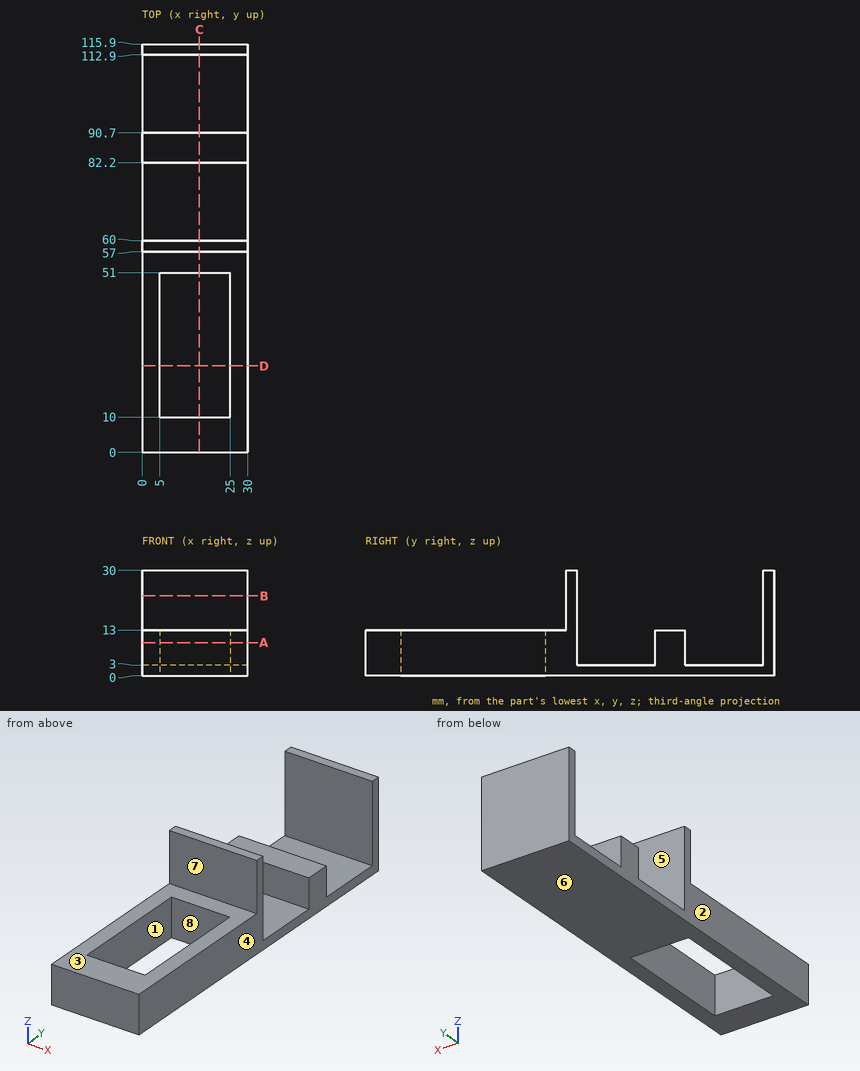
Geometry check sheet. Reference: drawing and pictorial views, mm from the part's lowest x, y, z. A direction names the side the tool comes from. Coordinates: 2 decimals unless noted, no trailing zeros. Order: outer loops, then holes, each group sorted by start corner. A loop starts at its lowest first (then second) coordinate and runs counter-clockwise, first axis right, second up.
Item 1: Section check C-C (x = 16.25). Enter the section's corners in (y, z).
Item 2: Scan lines: line 1 along Y through (x, z) = (19.75, 5.75); line 2 along Y through (x, z) = (27.5, 8); line 3 along Y through (x, z) = (19.75, 18.5). Record each from-to range of solid material in increasing order.
Item 3: Depth check by flat-ended pin: pin 1 (8 mm diameter, centred on x = 14, z = 18.5, fed in from -Y); pin 2 (6 mm diameter, centred on x = 7.5, y = 104.5, fed in from +Z); pin 3 (2.5 mm diameter, centred on x = 21, y = 85.5, fed in from +Z). Enter the tip coordinate at first touch or a pass-through.
Item 4: Section check A-A (z = 9.5). Enter the section's corners in (x, y), plus the area to 4 significant figures.
Item 5: Section check D-D (y = 24.5). Enter the section's corners in (x, z).
Item 6: Section check B-B (z = 22.75). Enter the section's corners in (x, y).
Item 7: Tool access check on the marked faces 5, 6, 7 and 8. Record the directions out of +Z, -Z, +X, -X, +Y, -Y that give a thin tool (end or side, any length) a straight path to the whole face; none if there is none.
Item 8: Mould release check, pull along X, two halves, no side actions. Record for the marked faces 1, 2, 3 and 4: released by +X, released by -X, zero draft, split by the parting line, or undercut.
Check sheet entries:
1. outline: (0, 0) - (10, 0) - (10, 13) - (0, 13) - close; (51, 0) - (115.9, 0) - (115.9, 30) - (112.9, 30) - (112.9, 3) - (90.7, 3) - (90.7, 13) - (82.2, 13) - (82.2, 3) - (60, 3) - (60, 30) - (57, 30) - (57, 13) - (51, 13) - close
2. line 1: y = 0 to 10, 51 to 60, 82.2 to 90.7, 112.9 to 115.9
2. line 2: y = 0 to 60, 82.2 to 90.7, 112.9 to 115.9
2. line 3: y = 57 to 60, 112.9 to 115.9
3. pin 1: stops at y = 57
3. pin 2: stops at z = 3
3. pin 3: stops at z = 13
4. outline: (0, 0) - (30, 0) - (30, 60) - (0, 60) - close; (0, 82.2) - (30, 82.2) - (30, 90.7) - (0, 90.7) - close; (0, 112.9) - (30, 112.9) - (30, 115.9) - (0, 115.9) - close; hole (5, 10) - (25, 10) - (25, 51) - (5, 51) - close
4. area: 1,325 mm2
5. outline: (0, 0) - (5, 0) - (5, 13) - (0, 13) - close; (25, 0) - (30, 0) - (30, 13) - (25, 13) - close
6. outline: (0, 57) - (30, 57) - (30, 60) - (0, 60) - close; (0, 112.9) - (30, 112.9) - (30, 115.9) - (0, 115.9) - close
7. face 5: +Z, +X, -X
7. face 6: -Z, +X, -X, +Y, -Y
7. face 7: +Z, +X, -X, -Y
7. face 8: +Z, -Z
8. face 1: undercut
8. face 2: released by -X
8. face 3: zero draft
8. face 4: released by +X
